Source: CAD feature listing. Evaluate the final solid. Frame: model axes, mm. Face numbers are marked on the shaded views. A direction names the side the tool comes from. Round coordinates to 2 decimals unless told otherwise and drop trailing zeros. Loops run counter-clockwise (first coordinate to the right, second up) from the corner with the lowest first, then second, coordinate; pieces in that order, holes last. Notation, with made-up numbers: M 22,27 L 58,27 A35 cw 58,62 Z; hole C 71.25,33.25 d10. An arc over 180 degrees is marked long. One line per item, written item: value.
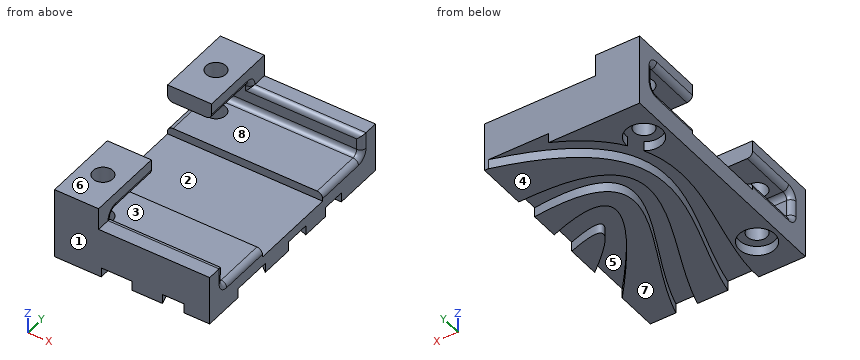
from build123d import *

# Parameters (mm, degrees)
BOSS_EXTRUDE1_DEPTH      = 11
BOSS_EXTRUDE1_DEPTH_BACK = 2
SKETCH1_W                = 28.18
SKETCH1_H                = 44
CUT_EXTRUDE1_DEPTH       = 37
SKETCH4_W                = 20.18
SKETCH4_H                = 4
CUT_EXTRUDE2_DEPTH       = 48
CUT_EXTRUDE3_DEPTH       = 1.75
SKETCH7_R                = 1.8
CUT_EXTRUDE4_DEPTH       = 23
FILLET1_R                = 1
SKETCH8_R                = 3.25
CUT_EXTRUDE5_DEPTH       = 1.75


with BuildPart() as part:
    # Sketch1 → Boss-Extrude1 (new, two sides: drawn at the far end of the back side and taken through both)
    with BuildSketch(Plane.XY.offset(-BOSS_EXTRUDE1_DEPTH_BACK)):
        Rectangle(SKETCH1_W, SKETCH1_H)
    extrude(amount=BOSS_EXTRUDE1_DEPTH + BOSS_EXTRUDE1_DEPTH_BACK)

    # Sketch3 → Cut-Extrude1 (cut)
    with BuildSketch(Plane.ZY.offset(14.09)):
        Polygon((8, 8), (11, 8), (11, -8), (8, -8), (8, -18.5), (3, -18.5), (3, -8), (1.5033938, -8), (1.5033938, 8), (3, 8), (3, 18.5), (8, 18.5), align=None)
    extrude(amount=-CUT_EXTRUDE1_DEPTH, mode=Mode.SUBTRACT)

    # Sketch4 → Cut-Extrude2 (cut)
    with BuildSketch(Plane.XZ.offset(22)):
        with Locations((4, 9)):
            Rectangle(SKETCH4_W, SKETCH4_H)
    extrude(amount=-CUT_EXTRUDE2_DEPTH, mode=Mode.SUBTRACT)

    # Sketch5 → Cut-Extrude3 (cut)
    with BuildSketch(Plane(origin=(0, 0, -2), x_dir=(-1, 0, 0), z_dir=(0, 0, -1))):
        with BuildLine():
            Line((-9.422350513, -22), (-5.513274624, -22))
            add(Edge.make_bspline(
                [(-14.09, 12.943541527), (17.027152303, 14.230895657), (-0.913223026, -5.637747584), (-5.513274624, -22)],
                knots=[0, 0, 0, 0, 0.88215351, 0.88215351, 0.88215351, 0.88215351], degree=3))
            Line((-14.09, 12.943541527), (-14.09, 8.727219843))
            add(Edge.make_bspline(
                [(-14.09, 8.727219843), (12.710361443, 11.678555955), (-5.250487577, -7.026945605), (-9.422350513, -22)],
                knots=[0, 0, 0, 0, 0.871233208, 0.871233208, 0.871233208, 0.871233208], degree=3))
        make_face()
        with BuildLine():
            add(Edge.make_bspline(
                [(-14.09, 3.523280295), (7.913446573, 11.6376574), (-14.09, -14.545652593)],
                knots=[0, 0, 0, 1, 1, 1], degree=2))
            Line((-14.09, 3.523280295), (-14.09, -1.131328535))
            add(Edge.make_bspline(
                [(-14.09, -1.131328535), (-1.654052468, 3.211926994), (-14.09, -7.240502624)],
                knots=[0, 0, 0, 1, 1, 1], degree=2))
            Line((-14.09, -7.240502624), (-14.09, -14.545652593))
        make_face()
        with BuildLine():
            add(Edge.make_bspline(
                [(-2.448223174, 22), (19.56705897, 11.536361781), (5.151599528, -7.62224079), (5.592236917, -22)],
                knots=[0, 0, 0, 0, 0.832841206, 0.832841206, 0.832841206, 0.832841206], degree=3))
            Line((-2.448223174, 22), (-13.413117725, 22))
            add(Edge.make_bspline(
                [(-13.413117725, 22), (18.496116363, 13.047461166), (3.546154763, -4.863207343), (0.001206333, -22)],
                knots=[0, 0, 0, 0, 0.886771983, 0.886771983, 0.886771983, 0.886771983], degree=3))
            Line((0.001206333, -22), (5.592236917, -22))
        make_face()
    extrude(amount=-CUT_EXTRUDE3_DEPTH, mode=Mode.SUBTRACT)

    # Sketch7 → Cut-Extrude4 (cut)
    with BuildSketch(Plane.XY.offset(11)):
        with Locations((-10.09, 15)):
            Circle(SKETCH7_R)
        with Locations((-10.09, -15)):
            Circle(SKETCH7_R)
    extrude(amount=-CUT_EXTRUDE4_DEPTH, mode=Mode.SUBTRACT)

    # Fillet1
    fillet1_edges = [part.edges().sort_by_distance(p)[0] for p in [
        (-14.09, -13.25, 3),
        (-14.09, -13.25, 8),
        (14.09, -13.25, 3),
        (-6.09, -13.25, 8),
        (14.09, 13.25, 3),
        (-14.09, 13.25, 3),
        (-14.09, 13.25, 8),
        (-6.09, 13.25, 8),
        (-14.09, -18.5, 5.5),
        (0, -18.5, 3),
        (14.09, -18.5, 5),
        (4, -18.5, 7),
        (-6.09, -18.5, 7.5),
        (-10.09, -18.5, 8),
        (14.09, 18.5, 5),
        (0, 18.5, 3),
        (-14.09, 18.5, 5.5),
        (-10.09, 18.5, 8),
        (-6.09, 18.5, 7.5),
        (4, 18.5, 7),
    ]]
    fillet(fillet1_edges, radius=FILLET1_R - 0.0001)  # a hair under: the kernel refuses the full size

    # Sketch8 → Cut-Extrude5 (cut)
    with BuildSketch(Plane(origin=(0, 0, -2), x_dir=(-1, 0, 0), z_dir=(0, 0, -1))):
        with Locations((10.09, -15)):
            Circle(SKETCH8_R)
        with Locations((10.09, 15)):
            Circle(SKETCH8_R)
    extrude(amount=-CUT_EXTRUDE5_DEPTH, mode=Mode.SUBTRACT)


solid = part.part
1. Section query C-C (y = -15). Count the separate pieces of the cut face and the enclosed holes in it, and give its area (3 significant figures).
Report:
separate pieces: 4
enclosed holes: 0
area: 116 mm2
2. Pin query (flat end, axial travel): pin 1 (10 mm diameter, centred on x = 10, y = 10.5, fed in from +Z); pin 2 (6 mm diameter, centred on x = -10.09, y = -15, fed in from -Z); pin 3 (6 mm diameter, centred on x = -10.09, y = 15, fed in from +Z); pin 4 (3 mm diameter, centred on x = 3.5, y = -21, fed in from +Z). Return the tip coordinate at first contact, or that it passes through.
Report:
pin 1: stops at z = 3
pin 2: stops at z = -0.25
pin 3: stops at z = 11
pin 4: stops at z = 7
3. Ray query, line 1 (Y direction, x = -10.09, z = 8.7); line 2 (Y direction, x = -10.09, z = -1.15); line 3 (Y direction, x = -10.09, z = 1.3). Return the intervals inside material, ascending. Write a range as [from, to].
Report:
line 1: y = [-22, -16.8], [-13.2, -8], [8, 13.2], [16.8, 22]
line 2: y = [-22, -18.25], [-11.75, 11.75], [18.25, 22]
line 3: y = [-22, -16.8], [-13.2, 13.2], [16.8, 22]
4. Section query B-B (z = 10). Return the cut outline in (x, y), and give its area (3 significant figures).
Report:
outline: M -14.09,-22 L -6.09,-22 L -6.09,-8 L -14.09,-8 Z; M -14.09,8 L -6.09,8 L -6.09,22 L -14.09,22 Z; hole C -10.09,-15 d3.6; hole C -10.09,15 d3.6
area: 204 mm2
5. Section query D-D (z = 0.75). Return the cut outline in (x, y).
Report:
outline: M -14.09,-22 L 14.09,-22 L 14.09,22 L -14.09,22 Z; hole C -10.09,-15 d3.6; hole C -10.09,15 d3.6
6. Section query A-A (z = 4.5). Return the cut outline in (x, y).
Report:
outline: M -14.09,-22 L 14.09,-22 L 14.09,-19.5 A1 ccw 13.09,-18.5 L -13.09,-18.5 A1 ccw -14.09,-19.5 Z; M -14.09,19.5 A1 ccw -13.09,18.5 L 13.09,18.5 A1 ccw 14.09,19.5 L 14.09,22 L -14.09,22 Z
7. Reachability of the marked faces 1, 2, 3, 4 and 5 from +Z, -Z, +X, -X, +Y, -Y: full face, straight path, thin tool, end or side. Return the list, or none.
Report:
face 1: +Z, -Z, +X, -X, -Y
face 2: +Z, +X, -X
face 3: +X, -X
face 4: -Z, +X, -X, +Y, -Y
face 5: -Z
8. Pull-direction query (Z, two-part tool) for the marked faces 6, 7 and 8; classes: released by +Z, released by -Z, zero draft, split by the parting line, or undercut.
Report:
face 6: released by +Z
face 7: released by -Z
face 8: undercut
